Autodesk Fusion 360 part; units mm, degrees
sketch "スケッチ1" plane through (0, 0, 0) normal (0, 0, 1) x (1, 0, 0)
  line L0 (0, 0) -> (29, 0)
  line L1 (29, 0) -> (29, 25.4)
  line L2 (29, 25.4) -> (0, 25.4)
  line L3 (0, 25.4) -> (0, 0)
  dimension "d1" = 29
  dimension "d2" = 25.4
extrude "押し出し2" add sketch "スケッチ1" along normal blind 12.7 makes body 1
sketch "スケッチ2" plane through (0, 0, 12.7) normal (0, 0, 1) x (-1, 0, 0)
  line L0 (0, -25.4) -> (0, 0)
  line L1 (0, 0) -> (-29, 0)
  line L2 (-29, 0) -> (-29, -25.4)
  line L3 (-29, -25.4) -> (0, -25.4)
  line L4 (-29, -12.7) -> (0, -12.7)
  line L5 (-14.5, -12.7) -> (-14.5, -25.4)
  line L6 (-14.5, 0) -> (-14.5, -12.7)
  line L7 (-14.5, -12.7) -> (-14.5, -22.48)
  circle A0 centre (-14.5, -22.48) radius 1.5
  circle A1 centre (-14.5, -2.92) radius 1.5
  dimension "d10" = 9.78
  dimension "d11" = 3
sketch "スケッチ3" plane through (29, 0, 0) normal (1, 0, 0) x (0, 1, 0)
  line L0 (0, 0) -> (25.4, 0)
  line L1 (25.4, 0) -> (25.4, 12.7)
  line L2 (25.4, 12.7) -> (0, 12.7)
  line L3 (0, 12.7) -> (0, 0)
  line L4 (22.4716, 12.7) -> (22.4716, 0)
  line L5 (2.9158, 12.7) -> (2.9158, 0)
  line L6 (0, 6.35) -> (25.4, 6.35)
  circle A0 centre (2.9158, 6.35) radius 1.5
  circle A1 centre (22.4716, 6.35) radius 1.5
  line L7 (12.7, 12.7) -> (12.7, 0)
  circle A2 centre (12.7, 6.35) radius 1.5
  dimension "d12" = 3
  dimension "d13" = 3
  dimension "d14" = 3
sketch "スケッチ4" plane through (0, 0, 0) normal (-1, 0, 0) x (0, -1, 0)
  line L0 (-25.4, 0) -> (0, 0)
  line L1 (0, 0) -> (0, 12.7)
  line L2 (0, 12.7) -> (-25.4, 12.7)
  line L3 (-25.4, 12.7) -> (-25.4, 0)
  line L4 (-22.4672, 12.7) -> (-22.4672, 0)
  line L5 (-2.918, 12.7) -> (-2.918, 0)
  line L6 (-25.4, 6.35) -> (0, 6.35)
  circle A0 centre (-22.4672, 6.35) radius 1.5
  circle A1 centre (-2.918, 6.35) radius 1.5
  dimension "d15" = 3
  dimension "d16" = 3
extrude "押し出し3" cut sketch "スケッチ4" against normal blind 9.144 contours L5 L6 A1 | L5 L6 A1 | L5 L6 A1 | L5 L6 A1 bodies 1
extrude "押し出し4" cut sketch "スケッチ4" against normal blind 9.144 contours L4 L6 A0 | L4 L6 A0 | L4 L6 A0 | L4 L6 A0 bodies 1
extrude "押し出し5" cut sketch "スケッチ2" against normal up to surface (12.7 mm away) contours L6 A1 | L6 A1 bodies 1
extrude "押し出し6" cut sketch "スケッチ2" against normal up to surface (12.7 mm away) contours L5 L7 A0 | L5 L7 A0 bodies 1
extrude "押し出し7" cut sketch "スケッチ3" against normal blind 9.144 contours L5 L6 A0 | L5 L6 A0 | L5 L6 A0 | L5 L6 A0 bodies 1
extrude "押し出し8" cut sketch "スケッチ3" against normal blind 9.144 contours L4 L6 A1 | L4 L6 A1 | L4 L6 A1 | L4 L6 A1 bodies 1
extrude "押し出し9" add sketch "スケッチ3" along normal blind 9.144 contours L6 L7 A2 | L6 L7 A2 | L6 L7 A2 | L6 L7 A2 bodies 1
copy_body "ボディ -> コンポーネント1" bodies 1 removing the originals makes body 2 in component "Component'"
extrude "押し出し1" [suppressed]
component "Component'" placed x (1, 0, 0) y (0, 1, 0) z (0, 0, 1) at (0, 0, 0)
Could you check a few things on this model? Use its own coordinates, in mm. A direction names the side the tool comes from. Round coordinates to 2 decimals unless told otherwise and drop trailing zeros. Loops run counter-clockwise (first coordinate to the right, second up) from the corner with the lowest first, then second, coordinate; pieces in that order, holes last. Notation, with made-up numbers: M 50.25,62 L 103.25,62 A19 ccw 103.25,93 Z; hole C -6.75,71.25 d5. An arc over 180 degrees is marked long. Put each result on its own line as item: value.
Q1. Imagine slicing it at A-A (y = 2.92). Write out the boundary of the cut face in (x, z), then the cut area to 3 significant figures.
Check result:
outline: M 0,0 L 13,0 L 13,12.7 L 0,12.7 L 0,7.85 L 9.14,7.85 L 9.14,4.85 L 0,4.85 Z; M 16,0 L 29,0 L 29,4.85 L 19.86,4.85 L 19.86,7.85 L 29,7.85 L 29,12.7 L 16,12.7 Z
area: 275 mm2
Q2. On a 3-axis mill with a long thin cutter (end or side, diameter ignored), from which of +Z, -Z, +X, -X, +Y, -Y can I reach the whole of each face in a straight line? I mean faces 4 (the face through (14, 0, 6)), 5 (the face through (24.492, 23.902, 6.801)), 6 (the face through (9.144, 3, 6)). Say none if no direction works.
Check result:
face 4: +Z, -Z, +X, -X, -Y
face 5: +X
face 6: -X
Q3. For pin 1 (2.5 mm diameter, centred on y = 2.92, z = 6.35, fed in from +X); pin 2 (1.5 mm diameter, centred on y = 8.5, z = 6, fed in from +X); pin 3 (2.5 mm diameter, centred on y = 22.47, z = 6.35, fed in from -X), each with a flat end and sliding along its axis, tell me the tip position at first contact or that it passes through.
Check result:
pin 1: x = 19.86
pin 2: x = 29
pin 3: x = 9.14
Q4. Thinking about a two-plate mould opening in Z: for faces 1 (the face through (19.856, 22, 6)), 2 (the face through (14, 13, 0)), 3 (the face through (33.508, 13.506, 5.085)), which applies, released by +Z, released by -Z, zero draft, split by the parting line, or undercut?
Check result:
face 1: undercut
face 2: released by -Z
face 3: split by the parting line
Q5. Imagine slicing it at C-C (z = 1). Write out the boundary of the cut face in (x, y).
Check result:
outline: M 0,0 L 29,0 L 29,25.4 L 0,25.4 Z; hole C 14.5,2.92 d3; hole C 14.5,22.48 d3
Q6. I need wall thicknesses on probe 1 along Y at (x, z) = (14.5, 6.75); probe 2 along X at (y, z) = (22.48, 9.5); probe 3 along X at (y, z) = (22.48, 6.25). Which ranges of each line are inside material? Lowest first, please.
Check result:
probe 1: 0 to 1.42, 4.42 to 20.98, 23.98 to 25.4
probe 2: 0 to 13, 16 to 29
probe 3: 9.14 to 13, 16 to 19.86
Q7. Imagine slicing it at D-D (y = 12.7). Write out the boundary of the cut face in (x, z).
Check result:
outline: M 0,0 L 29,0 L 29,4.85 L 38.14,4.85 L 38.14,7.85 L 29,7.85 L 29,12.7 L 0,12.7 Z
Q8. Imagine slicing it at B-B (x = 14.5). Write out the boundary of the cut face in (y, z).
Check result:
outline: M 0,0 L 1.42,0 L 1.42,12.7 L 0,12.7 Z; M 4.42,0 L 20.98,0 L 20.98,12.7 L 4.42,12.7 Z; M 23.98,0 L 25.4,0 L 25.4,12.7 L 23.98,12.7 Z
